The model under review builds one solid part; all positions refer to its coordinate system, in mm. Face numbers are marked on the shaded views. A direction names the side the tool comes from. Coordinates: 2 decimals unless noted, no trailing zeros. Loops run counter-clockwise (first coordinate to the right, second up) from the corner with the lowest first, then second, coordinate; pieces in that order, holes last. Notation, with made-up numbers: (-14, -29) - (-10, -29) arc R15 cw to (-10, -25) - close; hole circle Ø7 at (76, 54.25). An arc over 180 degrees is marked (long way). Answer in a Markdown table with one row per item. Add a question column.
(1) We need section D-D on x = 12. Write out the cut boundary in (y, z).
(2) We need section A-A on x = -42. Write out the cut boundary in (y, z), plus the area to 3 significant figures.
(3) For P1, Ø12, axis at x = -31, z = 17, coming from the -Y side; P2, Ø6, axis at y = -0.5, z = 14, coming from the -X side, all flat-tipped, find the tip position at first contact; note any pin that passes through.
(4) Machinability: for the marked faces 1 and 2, which of the approach directions +Z, -Z, +X, -X, +Y, -Y give a long, thin tool a straight path to every point of the face, cutting with its end or side? Answer none if there is none.
(5) We need section B-B on z = 2.75. Write out the cut boundary in (x, y), plus the area to 3 significant figures.
(6) For line 1 along Z through (x, y) = (-42, 38); line 2 along Y through (x, z) = (-41, 2); line 3 along Z through (x, y) = (-32, 38), list the stretches that pass through material, from the lowest coordinate up.
(7) We need section C-C on y = -8.5. Write out the cut boundary in (x, z).
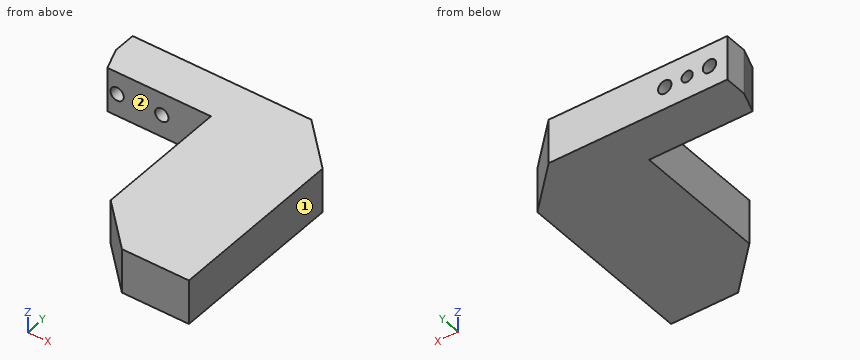
from build123d import *

# Parameters (mm, degrees)
SKETCH_1_W             = 100
SKETCH_1_H             = 100
EXTRUDE_1_DEPTH        = 20
MM_1_D                 = 6
MM_1_DEPTH             = 20
MM_1_TIP               = 1.802581857
HOLE_WIZARD_M6_1_D     = 5
HOLE_WIZARD_M6_1_DEPTH = 15
HOLE_WIZARD_M6_1_TIP   = 1.502151548
SKETCH_6_W             = 50
SKETCH_6_H             = 80
CUT_EXTRUDE_1_DEPTH    = 74.484692283
CHAMFER_1_SIZE         = 10
CHAMFER_1_SIZE2        = 3.639702343
CHAMFER_2_SIZE         = 20
CHAMFER_3_SIZE         = 20


with BuildPart() as part:
    # 草图1 → 凸台-拉伸1 (new body)
    with BuildSketch(Plane.XY):
        Rectangle(SKETCH_1_W, SKETCH_1_H)
    extrude(amount=EXTRUDE_1_DEPTH)

    # 大小mm 暗销孔1
    with Locations(Plane(origin=(0, 50, 0), x_dir=(1, 0, 0), z_dir=(0, 1, 0))):
        with Locations((-22, -10), (-42, -10)):
            Hole(MM_1_D / 2, depth=MM_1_DEPTH)
            with Locations((0, 0, -(MM_1_DEPTH + MM_1_TIP / 2))):  # 118° drill point
                Cone(0, MM_1_D / 2, MM_1_TIP, mode=Mode.SUBTRACT)

    # M6 螺纹孔1
    with Locations(Plane(origin=(0, 50, 0), x_dir=(1, 0, 0), z_dir=(0, 1, 0))):
        with Locations((-32, -10)):
            Hole(HOLE_WIZARD_M6_1_D / 2, depth=HOLE_WIZARD_M6_1_DEPTH)
            with Locations((0, 0, -(HOLE_WIZARD_M6_1_DEPTH + HOLE_WIZARD_M6_1_TIP / 2))):  # 118° drill point
                Cone(0, HOLE_WIZARD_M6_1_D / 2, HOLE_WIZARD_M6_1_TIP, mode=Mode.SUBTRACT)

    # 草图6 → 切除-拉伸1 (cut, through all)
    with BuildSketch(Plane(origin=(0, 0, 0), x_dir=(-1, 0, 0), z_dir=(0, 0, -1))):
        with Locations((25, -10)):
            Rectangle(SKETCH_6_W, SKETCH_6_H)
    extrude(amount=-CUT_EXTRUDE_1_DEPTH, mode=Mode.SUBTRACT)

    # 倒角1
    chamfer_1_edges = [part.edges().sort_by_distance(p)[0] for p in [
        (-50, 30, 10),
    ]]
    chamfer_1_side = [part.faces().sort_by_distance(p)[0] for p in [
        (-50, 40, 10),
    ]]
    chamfer(chamfer_1_edges, length=CHAMFER_1_SIZE, length2=CHAMFER_1_SIZE2, reference=chamfer_1_side[0])

    # 倒角2
    chamfer_2_edges = [part.edges().sort_by_distance(p)[0] for p in [
        (0, -50, 10),
    ]]
    chamfer(chamfer_2_edges, length=CHAMFER_2_SIZE)

    # 倒角3
    chamfer_3_edges = [part.edges().sort_by_distance(p)[0] for p in [
        (50, 50, 10),
    ]]
    chamfer(chamfer_3_edges, length=CHAMFER_3_SIZE)


solid = part.part
Outcome:
| question | item | result |
|---|---|---|
| 1 | outline | (-42, 0) - (50, 0) - (50, 20) - (-42, 20) - close |
| 2 | outline | (30, 0) - (50, 0) - (50, 7) - (30, 7) - close; (30, 13) - (50, 13) - (50, 20) - (30, 20) - close |
| 2 | area | 280 mm² |
| 3 | P1 | y = 30 |
| 3 | P2 | x = 0 |
| 4 | face 1 | +Z, -Z, +X, +Y, -Y |
| 4 | face 2 | +Z, -Z, -X, -Y |
| 5 | outline | (-50, 40) - (-46.36, 30) - (0, 30) - (0, -30) - (20, -50) - (50, -50) - (50, 30) - (30, 50) - (-50, 50) - close |
| 5 | area | 5,580 mm² |
| 6 | line 1 | 0 to 7, 13 to 20 |
| 6 | line 2 | 30 to 50 |
| 6 | line 3 | 0 to 7.5, 12.5 to 20 |
| 7 | outline | (0, 0) - (50, 0) - (50, 20) - (0, 20) - close |
